Here's how the part is built. I have some questions about the finished solid (model axes, mm). Face numbers are marked on the shaded views. A direction names the side the tool comes from. Give positions to 0.01 mm unless a question says otherwise; leave off trailing zeros. Loops run counter-clockwise (first coordinate to the right, second up) from the corner with the lowest first, then second, coordinate; pieces in that order, holes last.
Q1. For the marked faces 1 and 2, which set-ups out of +Z, -Z, +X, -X, +Y, -Y let a thin tool reach every point of the face, with its end or its side?
Q2. Suppose I cut it at A-A (z = 0). List the corners of the cut face in (x, y) for me, and give its area (3 significant figures).
Q3. I need wall thicknesses on probe 1 along Z at (x, y) = (-23, 0.25); probe 2 along X at (y, z) = (4, 2); probe 3 along Y at (x, z) = (-0.5, -0.5). Which ranges of each line are inside material? Lowest first, please.
Q4. Suppose I cut it at C-C (x = 0). List the corners of the cut face in (y, z) for me, and give its area (3 significant figures).
Q5. I'm going to push flat-ended pins straight in: P1, Ø1, axis at x = -10, y = -1, coming from the +Z side; P2, Ø8, axis at x = 17.5, y = 4, coming from the -Z side; P3, Ø12, axis at x = 27, z = -6.5, coming from the +Y side; P4, Ø8, axis at x = 16, y = 8, coming from the -Z side. Where does each tip first touch, or does it pass through?
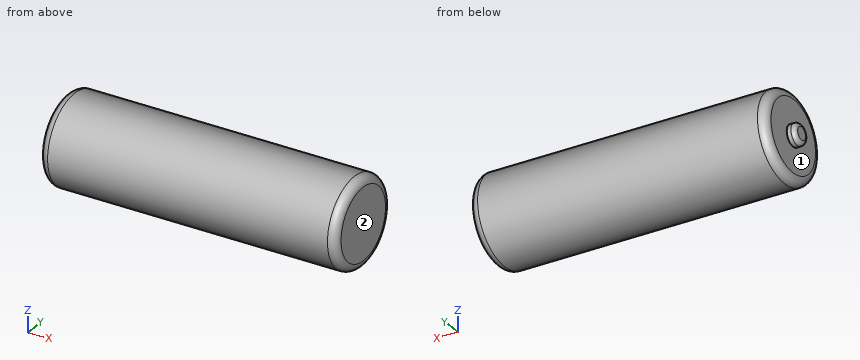
```python
from build123d import *

# Parameters (mm, degrees)
SKETCH_1_W      = 71
SKETCH_1_H      = 10.5
FILLET_1_R      = 2
FILLET_2_R      = 2
SKETCH_2_R      = 2.5
EXTRUDE_1_DEPTH = 2
FILLET_3_R      = 1


with BuildPart() as part:
    # 草图1 → 旋转3 (revolve)
    with BuildSketch(Plane(origin=(0, 0, 0), x_dir=(1, 0, 0), z_dir=(0, 1, 0))):
        with Locations((0, 5.25)):
            Rectangle(SKETCH_1_W, SKETCH_1_H)
    revolve(axis=Axis((35.5, 0, 0), (-1, 0, 0)))

    # 圆角1
    fillet_1_edges = [part.edges().sort_by_distance(p)[0] for p in [
        (-35.5, 0, 10.5),
    ]]
    fillet(fillet_1_edges, radius=FILLET_1_R)

    # 圆角2
    fillet_2_edges = [part.edges().sort_by_distance(p)[0] for p in [
        (35.5, 0, 10.5),
    ]]
    fillet(fillet_2_edges, radius=FILLET_2_R)

    # 草图2 → 凸台-拉伸1 (add)
    with BuildSketch(Plane.ZY.offset(35.5)):
        Circle(SKETCH_2_R)
    extrude(amount=EXTRUDE_1_DEPTH)

    # 圆角3
    fillet_3_edges = [part.edges().sort_by_distance(p)[0] for p in [
        (-37.5, 0, -2.5),
    ]]
    fillet(fillet_3_edges, radius=FILLET_3_R)


solid = part.part
```
Solutions:
1. face 1: -X
1. face 2: +Z, -Z, +X, +Y, -Y
2. outline: (-37.5, -1.5) arc R1 ccw to (-36.5, -2.5) - (-35.5, -2.5) - (-35.5, -8.5) arc R2 ccw to (-33.5, -10.5) - (33.5, -10.5) arc R2 ccw to (35.5, -8.5) - (35.5, 8.5) arc R2 ccw to (33.5, 10.5) - (-33.5, 10.5) arc R2 ccw to (-35.5, 8.5) - (-35.5, 2.5) - (-36.5, 2.5) arc R1 ccw to (-37.5, 1.5) - close
2. area: 1,500 mm2
3. probe 1: z = -10.5 to 10.5
3. probe 2: x = -35.5 to 35.5
3. probe 3: y = -10.49 to 10.49
4. outline: circle Ø21 at (0, 0)
4. area: 346 mm2
5. P1: stops at z = 10.49
5. P2: stops at z = -10.5
5. P3: stops at y = 10.49
5. P4: stops at z = -9.71
